CAD build for the part. Positions are in the model's coordinates, mm. Round coordinates to 2 decimals unless told otherwise and drop trailing zeros. Loops run counter-clockwise (first coordinate to the right, second up) from the corner with the lowest first, then second, coordinate; pieces in that order, holes last.
```python
from build123d import *

# Parameters (mm, degrees)
F1_DEPTH = 3
F2_W     = 5
F2_H     = 25
F3_DEPTH = 3.001
F4_R     = 2.5
F5_DEPTH = 3.001


with BuildPart() as f1:
    # F0 (on Front) → F1 (new body)
    with BuildSketch(Plane.XZ):
        with BuildLine():
            Line((-104.934193, 349.7432), (-334.934193, 349.7432))
            Line((-334.934193, 349.7432), (-334.934193, 299.7432))
            Line((-334.934193, 299.7432), (-134.934193, 299.7432))
            ThreePointArc((-134.934193, 299.7432), (-113.720989, 290.956403), (-104.934193, 269.7432))
            Line((-104.934193, 269.7432), (-104.934193, 19.7432))
            Line((-104.934193, 19.7432), (50.776976, -248.312824))
            Line((50.776976, -248.312824), (271.120743, -30.256354))
            Line((271.120743, -30.256354), (-104.934193, 349.7432))
        make_face()
    extrude(amount=F1_DEPTH)

    # F2 (on face) → F3 (cut, through all)
    with BuildSketch(Plane.XZ.offset(3)):
        with Locations((-302.434193, 327.2432)):
            Rectangle(F2_W, F2_H)
        with Locations((-177.434193, 327.2432)):
            Rectangle(F2_W, F2_H)
    extrude(amount=-F3_DEPTH, mode=Mode.SUBTRACT)

    # F4 (on face) → F5 (cut, through all)
    with BuildSketch(Plane.XZ.offset(3)):
        with Locations((228.694914, -30.035003)):
            Circle(F4_R)
        with Locations((242.763073, -44.25073)):
            Circle(F4_R)
        with Locations((50.998327, -205.886995)):
            Circle(F4_R)
        with Locations((65.066486, -220.102722)):
            Circle(F4_R)
    extrude(amount=-F5_DEPTH, mode=Mode.SUBTRACT)


solid = f1.part
```
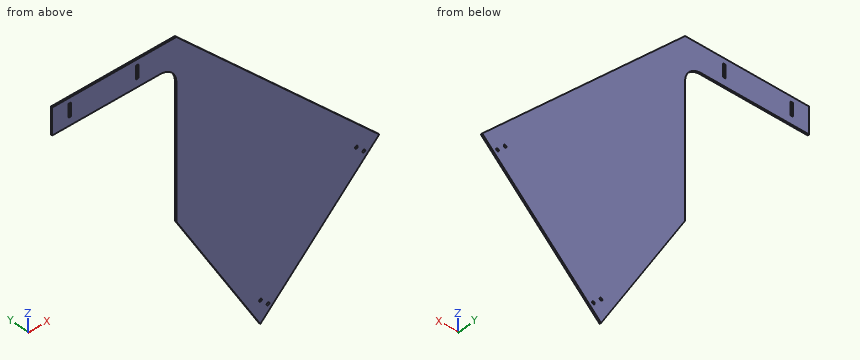
Item 1: Flat gauge pins, fed straight in: P1, Ø1.5, axis at x = -301.5, y = -2, coming from the -Z side; P2, Ø0.9, axis at y = -2, z = 323.5, coming from the +X side. Where does each tip first touch, or does it go through?
Answers follow:
P1: stops at z = 299.74
P2: stops at x = -78.52
Item 2: Cut at C-C, the plane x = -96.5. Give the cut face in (y, z), plus the area to 3 significant figures.
Answers follow:
outline: (-3, 5.22) - (0, 5.22) - (0, 341.22) - (-3, 341.22) - close
area: 1,010 mm2
Item 3: Probe line 1 (Z direction, x = -170, y = -0.9); line 2 (X direction, y = -2.35, z = -93); line 3 (Z direction, x = 169.5, y = -0.8). List the from-to ranges inside material, lowest first.
Answers follow:
line 1: z = 299.74 to 349.74
line 2: x = -39.44 to 207.72
line 3: z = -130.82 to 72.43
Item 4: Cut at A-A, the plane y = -2.3. Give the cut face in (x, z) (3 decimals), plus the area to 3 significant figures.
Answers follow:
outline: (-334.934, 299.743) - (-134.934, 299.743) arc R30 cw to (-104.934, 269.743) - (-104.934, 19.743) - (50.777, -248.313) - (271.121, -30.256) - (-104.934, 349.743) - (-334.934, 349.743) - close; hole (-304.934, 314.743) - (-299.934, 314.743) - (-299.934, 339.743) - (-304.934, 339.743) - close; hole (-179.934, 314.743) - (-174.934, 314.743) - (-174.934, 339.743) - (-179.934, 339.743) - close; hole circle Ø5 at (50.998, -205.887); hole circle Ø5 at (65.066, -220.103); hole circle Ø5 at (228.695, -30.035); hole circle Ø5 at (242.763, -44.251)
area: 120,000 mm2
Item 5: Cut at B-B, the plane z = 192. Give the cut face in (x, y).
Answers follow:
outline: (-104.93, -3) - (51.17, -3) - (51.17, 0) - (-104.93, 0) - close
